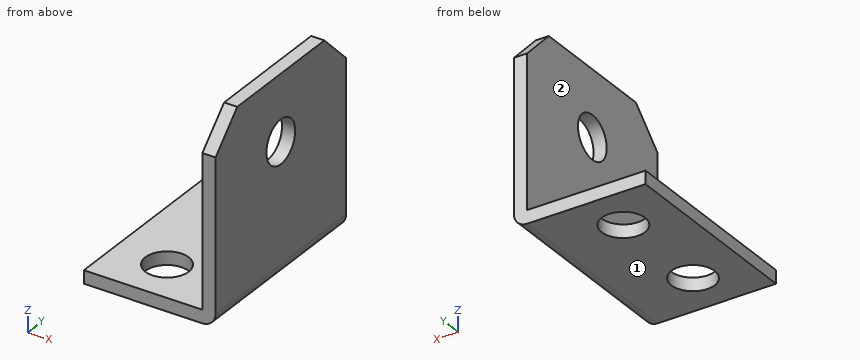
from build123d import *

# Parameters (mm, degrees)
F1_DEPTH = 30
F3_D     = 6.6
F5_D     = 6.6
F6_R     = 2
F7_SIZE  = 5


with BuildPart() as f1:
    # F0 (on Front) → F1 (new body)
    with BuildSketch(Plane.XZ):
        Polygon((-20, 0), (0, 0), (0, 30), (-2, 30), (-2, 2), (-20, 2), align=None)
    extrude(amount=F1_DEPTH)

    # F3 (through all)
    with Locations(Plane(origin=(0, 0, 0), x_dir=(1, 0, 0), z_dir=(0, 0, -1))):
        with Locations((-12, 23), (-12, 7)):
            Hole(F3_D / 2)

    # F5 (through all)
    with Locations(Plane.YZ):
        with Locations((-15, 20)):
            Hole(F5_D / 2)

    # F6
    f6_edges = [f1.edges().sort_by_distance(p)[0] for p in [
        (0, -15, 0),
    ]]
    fillet(f6_edges, radius=F6_R)

    # F7
    f7_edges = [f1.edges().sort_by_distance(p)[0] for p in [
        (-1, -30, 30),
        (-1, 0, 30),
    ]]
    chamfer(f7_edges, length=F7_SIZE)


solid = f1.part
Geometry check sheet. Reference: the model listing, model coordinates, mm. Face numbers are marked on the shaded views. A direction names the side the tool comes from. Round coordinates to 2 decimals unless told otherwise and drop trailing zeros. Write each loop counter-clockwise with the first axis right and the second up, starting at its lowest first coordinate (ties: lowest second). Pieces come first, ordered by that corner, then holes. Notation, with made-up numbers: (-30.5, 82.5) -> (-25.5, 82.5) arc R22 ccw to (-25.5, 107.5) -> close; hole circle Ø9 at (29.5, 68). An arc over 180 degrees is marked (long way). One line per item, written item: value. Start each with the question number.
(1) Access from +Z, -Z, +X, -X, +Y, -Y to the whole of each face (thin tool, end or side, straight path). Record for the marked faces 1 and 2.
(2) Cross-section at D-D, the plane y = -1.75. Record the cut outline in (x, z).
(3) Scan lines: line 1 (Y direction, x = -12, z = 0.75); line 2 (X direction, y = -9.75, z = 6.5); line 3 (Z direction, x = -13.25, y = -16.25). Record each from-to range of solid material in increasing order. Write a range as [from, to].
(4) Cross-section at C-C, the plane z = 20. Record the cut outline in (x, y).
(5) Go/stop test with flat-tipped pins: pin 1 Ø3 at (x, y) = (-13.5, -3.5) entering from +Z; pin 2 Ø8.5 at (y, z) = (-15, 20) entering from -X. Record where each tip stops, or that it passes through.
(6) Cross-section at B-B, the plane x = -12. Record the cut outline in (y, z), and give its area (3 significant figures).
(7) Cross-section at A-A, the plane y = -7. Record the cut outline in (x, z), and give its area (3 significant figures).
Answer:
1. face 1: -Z, +X, -X, +Y, -Y
1. face 2: +Z, -X, +Y, -Y
2. outline: (-20, 0) -> (-2, 0) arc R2 ccw to (0, 2) -> (0, 26.75) -> (-2, 26.75) -> (-2, 2) -> (-20, 2) -> close
3. line 1: [-30, -26.3], [-19.7, -10.3], [-3.7, 0]
3. line 2: [-2, 0]
3. line 3: [0, 2]
4. outline: (-2, -30) -> (0, -30) -> (0, -18.3) -> (-2, -18.3) -> close; (-2, -11.7) -> (0, -11.7) -> (0, 0) -> (-2, 0) -> close
5. pin 1: z = 2
5. pin 2: x = -2
6. outline: (-30, 0) -> (-26.3, 0) -> (-26.3, 2) -> (-30, 2) -> close; (-19.7, 0) -> (-10.3, 0) -> (-10.3, 2) -> (-19.7, 2) -> close; (-3.7, 0) -> (0, 0) -> (0, 2) -> (-3.7, 2) -> close
6. area: 33.6 mm²
7. outline: (-20, 0) -> (-15.3, 0) -> (-15.3, 2) -> (-20, 2) -> close; (-8.7, 0) -> (-2, 0) arc R2 ccw to (0, 2) -> (0, 30) -> (-2, 30) -> (-2, 2) -> (-8.7, 2) -> close
7. area: 81.9 mm²
